Geometry check sheet. Reference: drawing and pictorial views, mm from the part's lowest x, y, z. Round coordinates to 2 decimals unless told otherwise and drop trailing zeros. Write each loop counter-clockwise with the first axis right and the second up, starting at its lowest first coordinate (ties: lowest second). Pieces come first, ordered by that corner, then holes. Notation, with made-up numbers: M 63.25,-10 L 115.25,-10 A23 cw 115.25,3 Z; hole C 58.25,61 d6. An arc over 180 degrees is marked long. Put each result on its own line as item: value. Start each with the question number.
(1) Section check B-B on x = 3. Record the cut outline in (y, z).
(2) Section check C-C on y = 15. Record the cut outline in (x, z).
(3) Material ranges on probe 1 along Y at (x, z) = (4.55, 3); probe 2 along Y at (x, z) = (3, 1.2); probe 3 along Y at (x, z) = (3, 2.55), recorded low to high.
(4) Section check D-D on x = 4.9. Record the cut outline in (y, z), then the cut area to 3 significant figures.
(5) Section check A-A on z = 3.75. Record the cut outline in (x, y), then the cut area to 3 significant figures.
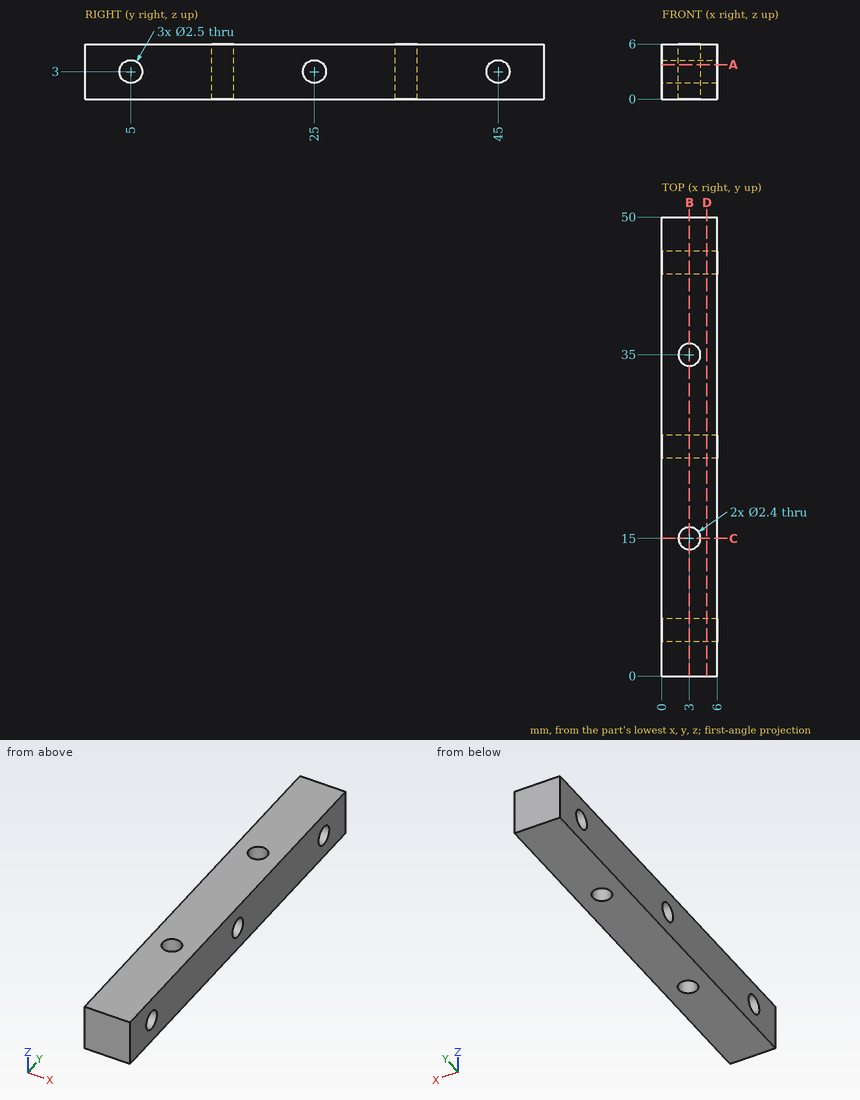
Answers follow:
1. outline: M 0,0 L 13.8,0 L 13.8,6 L 0,6 Z; M 16.2,0 L 33.8,0 L 33.8,6 L 16.2,6 Z; M 36.2,0 L 50,0 L 50,6 L 36.2,6 Z; hole C 5,3 d2.5; hole C 25,3 d2.5; hole C 45,3 d2.5
2. outline: M 0,0 L 1.8,0 L 1.8,6 L 0,6 Z; M 4.2,0 L 6,0 L 6,6 L 4.2,6 Z
3. probe 1: y = 0 to 3.75, 6.25 to 23.75, 26.25 to 43.75, 46.25 to 50
3. probe 2: y = 0 to 13.8, 16.2 to 33.8, 36.2 to 50
3. probe 3: y = 0 to 3.83, 6.17 to 13.8, 16.2 to 23.83, 26.17 to 33.8, 36.2 to 43.83, 46.17 to 50
4. outline: M 0,0 L 50,0 L 50,6 L 0,6 Z; hole C 5,3 d2.5; hole C 25,3 d2.5; hole C 45,3 d2.5
4. area: 285 mm^2
5. outline: M 0,0 L 6,0 L 6,4 L 0,4 Z; M 0,6 L 6,6 L 6,24 L 0,24 Z; M 0,26 L 6,26 L 6,44 L 0,44 Z; M 0,46 L 6,46 L 6,50 L 0,50 Z; hole C 3,15 d2.4; hole C 3,35 d2.4
5. area: 255 mm^2
